Geometry: see drawing. Coordinates: mm, zero at the bounding-box minimum. A direction names the side the tool comes from. Give positions to 0.01 mm unless a question says otherwise; leave off trailing zeros. Write each loop counter-clockwise with the first axis right and the second up, starting at its lowest first coordinate (ties: lowest second). Pieces come first, ordered by that corner, then holes. Notation, with made-up numbers: (43, -25) - (67, -25) arc R12 ccw to (67, -18) - close; hole circle Ø2 at (53.5, 30). An arc over 180 degrees is marked (long way). Return JSON: item names as keys, results as strings.
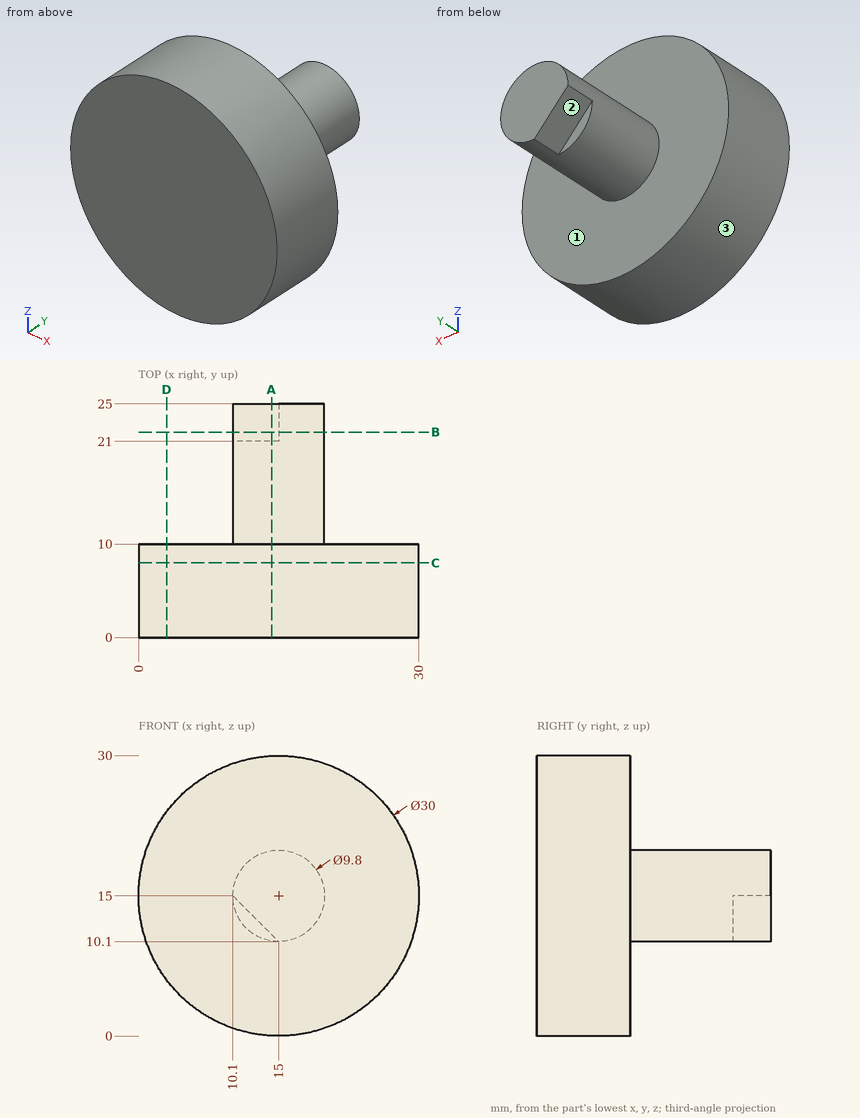
Q1. Section query C-C, the plane y = 8. Return the cut outline in (x, z).
Answer key:
{"outline": "circle Ø30 at (15, 15)"}
Q2. Set-up query: the marked faces 1, 2 and 3. Return all of +Z, -Z, +X, -X, +Y, -Y with unobstructed straight access to the full face (end or side cutting, diameter ignored); none if empty.
Answer key:
{"face 1": "+Y", "face 2": "-Z, -X, +Y", "face 3": "+Y, -Y"}
Q3. Section query D-D, the plane x = 3. Return the cut outline in (y, z), plus the area to 3 significant figures.
Answer key:
{"outline": "(0, 6) - (10, 6) - (10, 24) - (0, 24) - close", "area": "180 mm^2"}
Q4. Section query A-A, the plane x = 14.25. Return the cut outline in (y, z).
Answer key:
{"outline": "(0, 0.02) - (10, 0.02) - (10, 10.16) - (21, 10.16) - (21, 10.85) - (25, 10.85) - (25, 19.84) - (10, 19.84) - (10, 29.98) - (0, 29.98) - close"}
Q5. Material intervals for probe 1 along Y at (x, z) = (7.75, 17.5); probe 2 along X at (y, z) = (6.75, 3.25); probe 3 along Z at (x, y) = (5.25, 2), sorted ascending. Write a range as [from, to].
Answer key:
{"probe 1": "y = [0, 10]", "probe 2": "x = [5.68, 24.32]", "probe 3": "z = [3.6, 26.4]"}
Q6. Pin query (flat end, axial travel): P1, Ø8, axis at y = 12, z = 4, coming from the -X side; P2, Ø1, axis at y = 8, z = 6, coming from the +X side; P3, Ø4, axis at y = 21.5, z = 15, coming from the +X side. Return the tip coordinate at first contact, or that it passes through.
Answer key:
{"P1": "stops at x = 2.03", "P2": "stops at x = 27.36", "P3": "stops at x = 19.9"}
Q7. Section query B-B, the plane y = 22. Return the cut outline in (x, z).
Answer key:
{"outline": "(10.1, 15) - (15, 10.1) arc R4.9 ccw (long way) to start"}
